Geometry check sheet. Reference: the model listing, model coordinates, mm. Round coordinates to 2 decimals unless told otherwise and drop trailing zeros. Order: outer loops, then holes, each group sorted by start corner. A loop starts at its lowest first (then second) coordinate and runs counter-clockwise, first axis right, second up. Notation, with made-up numbers: (48.25, 54.5) - (102.25, 54.5) arc R17 ccw to (102.25, 78.5) - close; hole circle Ø4 at (-33.5, -22). An arc over 180 degrees is marked (long way). Return JSON: item names as keys, results as strings. Group by question number.
Q1. Sectioned sample at B-B, the plane y = -43. Record the cut outline in (x, z), then the cut area to 3 significant figures.
Q2. Material ranges on line 1 along Y through (x, z) = (123, 9.9); line 2 along X through (y, z) = (18.5, 9.55); line 3 along X through (y, z) = (0.5, 8.8), recorded low to high.
Q3. Gauge pin test, flat ends, axial feed: pin 1 Ø2 at (x, y) = (-11.31, -11.31) entering from -Z; pin 2 Ø1.5 at (x, z) = (2, 10.5) entering from -Y; pin 3 Ø4 at (x, y) = (77, -43) entering from +Z; pin 4 Ø1.2 at (y, z) = (19.5, 9.5) entering from -X. Record the tip position at first contact, or that the pin passes through.
Q4. Sectioned sample at C-C, the plane x = 0. Record the cut outline in (y, z).
Q5. Sectioned sample at A-A, the plane x = 123. Record the cut outline in (y, z), then the cut area to 3 significant figures.
Q6. Sectioned sample at D-D, the plane y = 0. Record the cut outline in (x, z), then the cut area to 3 significant figures.
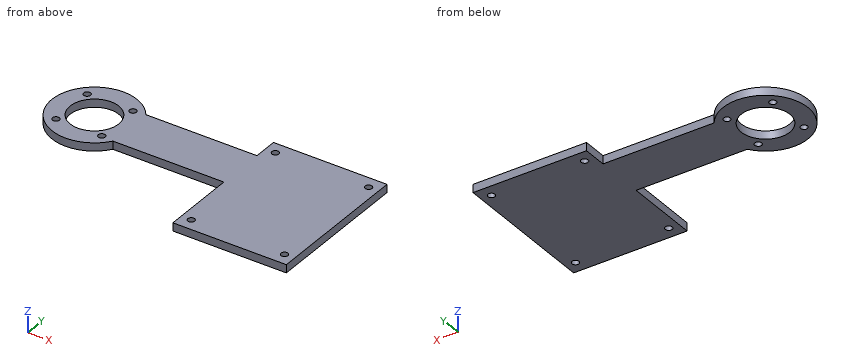
Solid Edge part; units mm, degrees
sketch "Sketch1" plane through (0, 0, 8) normal (0, 0, 1) x (1, 0, 0)
  circle A0 centre (0, 0) radius 21
  circle A1 centre (0, 0) radius 12
  circle A2 centre (11.3137, 11.3137) radius 1.7
  circle A3 centre (-11.3137, 11.3137) radius 1.7
  circle A4 centre (-11.3137, -11.3137) radius 1.7
  circle A5 centre (11.3137, -11.3137) radius 1.7
extrude "ExtrudedProtrusion_1" add sketch "Sketch1" along normal blind 4
sketch "Sketch2" plane through (0, 0, 8) normal (0, 0, 1) x (1, 0, 0)
  line L0 (12, -12) -> (88, -12)
  line L1 (88, -12) -> (88, 12)
  line L2 (88, 12) -> (12, 12)
  line L3 (12, 12) -> (12, -12)
extrude "ExtrudedProtrusion_2" add sketch "Sketch2" along normal blind 4
sketch "Sketch3" plane through (0, 0, 8) normal (0, 0, 1) x (1, 0, 0)
  line L0 (72, -49) -> (128, -49)
  line L1 (128, -49) -> (128, 24)
  line L2 (128, 24) -> (72, 24)
  line L3 (72, 24) -> (72, -49)
  circle A0 centre (77, -43) radius 1.7
  circle A1 centre (123, -43) radius 1.7
  circle A2 centre (77, 18) radius 1.7
  circle A3 centre (123, 18) radius 1.7
extrude "ExtrudedProtrusion_3" add sketch "Sketch3" along normal blind 4
sketch "Sketch4" plane through (0, 0, 8) normal (0, 0, 1) x (1, 0, 0)
  circle A0 centre (11.3137, 11.3137) radius 1.7
  circle A1 centre (-11.3137, 11.3137) radius 1.7
  circle A2 centre (-11.3137, -11.3137) radius 1.7
  circle A3 centre (11.3137, -11.3137) radius 1.7
  circle A4 centre (77, -43) radius 1.7
  circle A5 centre (123, -43) radius 1.7
  circle A6 centre (77, 18) radius 1.7
  circle A7 centre (123, 18) radius 1.7
extrude "ExtrudedCutout_1" cut sketch "Sketch4" along normal blind 4
Reply:
{
 "1": {"outline": "(72, 8) - (75.3, 8) - (75.3, 12) - (72, 12) - close; (78.7, 8) - (121.3, 8) - (121.3, 12) - (78.7, 12) - close; (124.7, 8) - (128, 8) - (128, 12) - (124.7, 12) - close", "area": "197 mm^2"},
 "2": {"line 1": "-49 to -44.7, -41.3 to 16.3, 19.7 to 24", "line 2": "-9.94 to 9.94, 72 to 75.38, 78.62 to 121.38, 124.62 to 128", "line 3": "-20.99 to -11.99, 11.99 to 128"},
 "3": {"pin 1": "through", "pin 2": "y = -20.96", "pin 3": "z = 12", "pin 4": "x = -9.15"},
 "4": {"outline": "(-21, 8) - (-12, 8) - (-12, 12) - (-21, 12) - close; (12, 8) - (21, 8) - (21, 12) - (12, 12) - close"},
 "5": {"outline": "(-49, 8) - (-44.7, 8) - (-44.7, 12) - (-49, 12) - close; (-41.3, 8) - (16.3, 8) - (16.3, 12) - (-41.3, 12) - close; (19.7, 8) - (24, 8) - (24, 12) - (19.7, 12) - close", "area": "265 mm^2"},
 "6": {"outline": "(-21, 8) - (-12, 8) - (-12, 12) - (-21, 12) - close; (12, 8) - (128, 8) - (128, 12) - (12, 12) - close", "area": "500 mm^2"}
}
